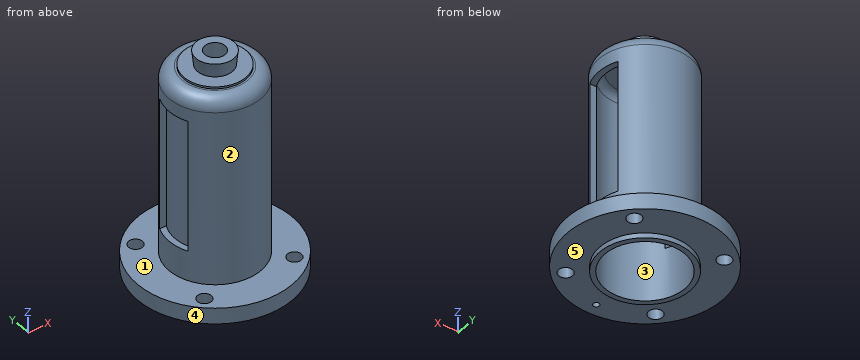
from build123d import *

# Parameters (mm, degrees)
F5_D          = 20.376
F7_D          = 14
F8_W          = 38
F8_H          = 132
F9_DEPTH      = 77.501
F9_DEPTH_BACK = 77.501
F11_D         = 6
F11_DEPTH     = 10
F11_TIP       = 1.8025818571


with BuildPart() as f1:
    # F0 (on Right) → F1 (revolve)
    with BuildSketch(Plane.YZ):
        with BuildLine():
            Line((19, 225), (0, 225))
            Line((0, 225), (0, 0))
            Line((0, 0), (45, 0))
            Line((45, 0), (45, 5))
            Line((45, 5), (77.5, 5))
            Line((77.5, 5), (77.5, 21))
            Line((77.5, 21), (46, 21))
            Line((46, 21), (46, 196))
            ThreePointArc((46, 196), (42.1923881554, 205.1923881554), (33, 209))
            Line((33, 209), (31, 209))
            Line((31, 209), (31, 211))
            Line((31, 211), (17.5, 211))
            Line((17.5, 211), (19, 225))
        make_face()
    revolve(axis=Axis((0, 0, 103.9262376726), (0, 0, -1)))

    # F2 (on Right) → F3 (revolve, cut)
    with BuildSketch(Plane.YZ):
        with BuildLine():
            Line((33, 203), (0, 203))
            Line((0, 203), (0, -6))
            Line((0, -6), (40, -6))
            Line((40, -6), (40, 196))
            ThreePointArc((40, 196), (37.9497474683, 200.9497474683), (33, 203))
        make_face()
    revolve(axis=Axis((0, 0, 103.9262376726), (0, 0, -1)), mode=Mode.SUBTRACT)

    # F5 (through all)
    with Locations(Plane.XY.offset(225)):
        with Locations((0, 0)):
            Hole(F5_D / 2)

    # F7 (through all)
    with Locations(Plane.XY.offset(21)):
        with Locations((45.9619407771, 45.9619407771), (45.9619407771, -45.9619407771), (-45.9619407771, 45.9619407771), (-45.9619407771, -45.9619407771)):
            Hole(F7_D / 2)

    # F8 (on Right) → F9 (cut, two sides)
    with BuildSketch(Plane.YZ) as f9_sk:
        with Locations((0, 117)):
            Rectangle(F8_W, F8_H)
    extrude(amount=-F9_DEPTH, mode=Mode.SUBTRACT)
    extrude(f9_sk.sketch, amount=F9_DEPTH_BACK, mode=Mode.SUBTRACT)

    # F11
    with Locations(Plane(origin=(0, 0, 5), x_dir=(1, 0, 0), z_dir=(0, 0, -1))):
        with Locations((0, 65)):
            Hole(F11_D / 2, depth=F11_DEPTH)
            with Locations((0, 0, -(F11_DEPTH + F11_TIP / 2))):  # 118° drill point
                Cone(0, F11_D / 2, F11_TIP, mode=Mode.SUBTRACT)


solid = f1.part
Design review of the part built by this model. Coordinates are the model's own, in mm. Face numbers are marked on the shaded views. A direction names the side the tool comes from. Coordinates: 2 decimals unless noted, no trailing zeros. Order: outer loops, then holes, each group sorted by start corner. A loop starts at its lowest first (then second) coordinate and runs counter-clockwise, first axis right, second up. Notation, with made-up numbers: (79.25, -25.75) -> (96.25, -25.75) arc R36 cw to (96.25, 11.25) -> close; hole circle Ø8 at (76.5, 46.5). An arc over 180 degrees is marked (long way). One line per item, written item: value.
1) We need section B-B, the plane y = 0. Count the separate pieces of the cut face and the enclosed holes in it, then the cut area to 3 significant figures.
Output values:
separate pieces: 4
enclosed holes: 0
area: 2,540 mm2
2) We need section A-A, the plane z = 147.5. Give the boundary of the cut face in (x, y), then the cut area to 3 significant figures.
Output values:
outline: (-41.89, -19) arc R46 ccw to (41.89, -19) -> (35.2, -19) arc R40 cw to (-35.2, -19) -> close; (-41.89, 19) -> (-35.2, 19) arc R40 cw to (35.2, 19) -> (41.89, 19) arc R46 ccw to start
area: 1,150 mm2
3) To check wall thickness, follow probe 1 along Y at (x, z) = (2, 25.5); probe 2 along Z at (x, y) = (45, 30); probe 3 along Z at (x, y) = (-20.5, 12). State the ranges of each line that lie inside material, in increasing order. Write a range as [from, to].
Output values:
probe 1: y = [-45.96, -39.95], [39.95, 45.96]
probe 2: z = [5, 21]
probe 3: z = [203, 211]
4) We need section D-D, the plane y = 64. Give the boundary of the cut face in (x, z).
Output values:
outline: (-43.71, 5) -> (43.71, 5) -> (43.71, 21) -> (-43.71, 21) -> close
5) We need section C-C, the plane z = 40. Give the boundary of the cut face in (x, y).
Output values:
outline: circle Ø92 at (0, 0); hole circle Ø80 at (0, 0)
6) Draft analysis for pull direction X (two halves, no side actions). For the marked faces 1, 2 and 3, state which applies: +X half, -X half, draft (parallel to the pull), parting line (faces both ways), or undercut.
Output values:
face 1: draft
face 2: parting line
face 3: undercut
7) Machinability: for the marked faces 4 and 5, which of the approach directions +Z, -Z, +X, -X, +Y, -Y give a long, thin tool a straight path to every point of the face, cutting with its end or side? Answer none if there is none.
Output values:
face 4: +Z, -Z
face 5: -Z
8) Clearance check with flat-ended pins moving along their axes: P1, Ø18, axis at x = -45.96, y = 45.96, coming from the +Z side; P2, Ø6, axis at x = -34, z = 48.5, coming from the +Y side; P3, Ø5.5, axis at x = -37, z = 108.5, coming from the -Y side; P4, Ø8, axis at x = 4.5, y = -38.5, coming from the -Z side. State where each tip first meets the part, or that it passes through.
Output values:
P1: stops at z = 21
P2: stops at y = 33.99
P3: stops at y = -30.71
P4: stops at z = 0
